Here's how the part is built. I have some questions about the finished solid (model axes, mm). A direction names the side the tool comes from. Coordinates: 2 decimals unless noted, no trailing zeros. Loops run counter-clockwise (first coordinate to the right, second up) from the corner with the lowest first, then second, coordinate; pieces in that order, holes last.
from build123d import *

# Parameters (mm, degrees)
SKETCH_R        = 11
PAD_DEPTH       = 6.6
SKETCH001_R     = 11
SKETCH001_R_2   = 6
POCKET_DEPTH    = 4.3
POCKET001_DEPTH = 6.601
SKETCH003_W     = 1.7
SKETCH003_H     = 1.7
PAD001_DEPTH    = 3
SKETCH004_W     = 2
SKETCH004_H     = 2
POCKET002_DEPTH = 4.3


with BuildPart() as part:
    # Sketch → Pad (new body)
    with BuildSketch(Plane.XY):
        Circle(SKETCH_R)
    extrude(amount=PAD_DEPTH)

    # Sketch001 → Pocket (cut)
    with BuildSketch(Plane(origin=(0, 0, 0), x_dir=(1, 0, 0), z_dir=(0, 0, -1))):
        Circle(SKETCH001_R)
        Circle(SKETCH001_R_2, mode=Mode.SUBTRACT)
    extrude(amount=-POCKET_DEPTH, mode=Mode.SUBTRACT)

    # Sketch002 → Pocket001 (cut, through all)
    with BuildSketch(Plane.XY.offset(6.6)):
        with BuildLine():
            Line((-2.683282, 0.8), (2.683282, 0.8))
            ThreePointArc((-2.683282, 0.8), (0, -2.8), (2.683282, 0.8))
        make_face()
    extrude(amount=-POCKET001_DEPTH, mode=Mode.SUBTRACT)

    # Sketch003 → Pad001 (new body)
    with BuildSketch(Plane(origin=(0, 0, 0), x_dir=(1, 0, 0), z_dir=(0, 0, -1))):
        with Locations((0, 4.35)):
            Rectangle(SKETCH003_W, SKETCH003_H)
        with Locations((0, -4.35)):
            Rectangle(SKETCH003_W, SKETCH003_H)
    extrude(amount=PAD001_DEPTH)

    # Sketch004 → Pocket002 (cut)
    with BuildSketch(Plane(origin=(0, 0, 0), x_dir=(1, 0, 0), z_dir=(0, 0, -1))):
        with Locations((-4.2, 0)):
            Rectangle(SKETCH004_W, SKETCH004_H)
        with Locations((4.2, 0)):
            Rectangle(SKETCH004_W, SKETCH004_H)
    extrude(amount=-POCKET002_DEPTH, mode=Mode.SUBTRACT)


solid = part.part
Q1. Suppose I cut it at B-B on z = 1. Write out the boundary of the cut face in (x, y), and give its area (3 significant figures).
Q2. Suppose I cut it at C-C on y = 0. Write out the boundary of the cut face in (x, z).
Q3. Suppose I cut it at A-A on x = 0. Write out the boundary of the cut face in (y, z).
Q4. We'd pull the mould along X, two halves only. Please class faces 1 (the flat face through (4, 1, 2)), 2 (the flat face through (0.85, 4, -1)), 3 (the flat face through (-0.85, -4, -1)), 4 (the flat face through (0, -4, -3)): pulls with the +X half, pulls with the -X half, needs draft (parallel to the pull), parting line crosses it, or undercut.
Q5. For faces 5 (the flat face through (0, 3.5, -1)), 6 (the flat face through (-3.2, 0, 2)), 7 (the flat face through (0, -5.2, -1)), 8 (the flat face through (0, 5.2, -1)), 9 (the flat face through (-0.85, 4, -1)), which set-ups out of +Z, -Z, +X, -X, +Y, -Y let a thin tool reach every point of the face, with its end or its side?
Q6. Please list where these lines run through material, in increasing order: probe 1 along X at (y, z) = (0, 1.5); probe 2 along Y at (x, z) = (0, 4.75); probe 3 along Y at (x, z) = (0, 4).
Q7. Will these pins go through, and if not, where does the flat tip stop? P1, Ø0.6, axis at y = 0, z = 3, coming from the -X side; P2, Ø3, axis at y = -5, z = 5.5, coming from the -X side; P3, Ø1.6, axis at y = -0.5, z = 1.5, coming from the +X side; P4, Ø4.5, axis at x = -0.5, z = 4, coming from the -Y side.
Q8. Suppose I cut it at D-D on z = 5.75. Write out the boundary of the cut face in (x, y), and give its area (3 significant figures).
Check values:
1. outline: circle Ø12 at (0, 0); hole (-5.2, -1) - (-3.2, -1) - (-3.2, 1) - (-5.2, 1) - close; hole (-2.68, 0.8) arc R2.8 ccw (long way) to (2.68, 0.8) - close; hole (3.2, -1) - (5.2, -1) - (5.2, 1) - (3.2, 1) - close
1. area: 88.4 mm2
2. outline: (-11, 4.3) - (-6, 4.3) - (-6, 0) - (-5.2, 0) - (-5.2, 4.3) - (-3.2, 4.3) - (-3.2, 0) - (-2.8, 0) - (-2.8, 6.6) - (-11, 6.6) - close; (2.8, 0) - (3.2, 0) - (3.2, 4.3) - (5.2, 4.3) - (5.2, 0) - (6, 0) - (6, 4.3) - (11, 4.3) - (11, 6.6) - (2.8, 6.6) - close
3. outline: (-11, 4.3) - (-6, 4.3) - (-6, 0) - (-5.2, 0) - (-5.2, -3) - (-3.5, -3) - (-3.5, 0) - (-2.8, 0) - (-2.8, 6.6) - (-11, 6.6) - close; (0.8, 0) - (3.5, 0) - (3.5, -3) - (5.2, -3) - (5.2, 0) - (6, 0) - (6, 4.3) - (11, 4.3) - (11, 6.6) - (0.8, 6.6) - close
4. face 1: undercut
4. face 2: pulls with the +X half
4. face 3: pulls with the -X half
4. face 4: needs draft
5. face 5: -Z, +X, -X
5. face 6: -Z
5. face 7: -Z, +X, -X, -Y
5. face 8: -Z, +X, -X, +Y
5. face 9: -Z, -X, +Y, -Y
6. probe 1: x = -6 to -5.2, -3.2 to -2.8, 2.8 to 3.2, 5.2 to 6
6. probe 2: y = -11 to -2.8, 0.8 to 11
6. probe 3: y = -6 to -2.8, 0.8 to 6
7. P1: stops at x = -6
7. P2: stops at x = -10.43
7. P3: stops at x = 6
7. P4: stops at y = -11
8. outline: circle Ø22 at (0, 0); hole (-2.68, 0.8) arc R2.8 ccw (long way) to (2.68, 0.8) - close
8. area: 363 mm2
